from build123d import *

# Parameters (mm, degrees)
SV_DEPTH           = 9
SKETCH3_W          = 35.897762959
SKETCH3_H          = 1.597828601
CUT_EXTRUDE1_DEPTH = 3.5


with BuildPart() as part:
    # Sketch1 → SV (new body)
    with BuildSketch(Plane(origin=(0, 0, 0), x_dir=(1, 0, 0), z_dir=(0, 1, 0))):
        Polygon((-20.189, 2.5), (21.25, 2.5), (21.25, -1.44), (21.25, -2.5), (20.19, -2.5), (-21.25, -2.5), (-21.25, 1.439), align=None)
    extrude(amount=SV_DEPTH)

    # Sketch3 → Cut-Extrude1 (cut)
    with BuildSketch(Plane(origin=(0, 9, 0), x_dir=(1, 0, 0), z_dir=(0, 1, 0))):
        Polygon((-20.202517392, 0.734832739), (-18.867516597, 0.734832739), (-18.867516597, 1.51327079), (19.169882457, 1.51327079), (19.169882457, 0.573528463), (20.36118295, 0.573528463), (20.36118295, -1.024300139), (19.169882457, -1.024300139), (19.169882457, -1.572342426), (-18.867516597, -1.572342426), (-18.867516597, -0.862995862), (-20.202517392, -0.862995862), align=None)
        with Locations((0.304154287, -0.064081561)):
            Rectangle(SKETCH3_W, SKETCH3_H, mode=Mode.SUBTRACT)
    extrude(amount=-CUT_EXTRUDE1_DEPTH, mode=Mode.SUBTRACT)


solid = part.part
Input: part model. Units: mm. Frame: model coordinates. A direction names the side the tool comes from. Round coordinates to 2 decimals unless told otherwise and drop trailing zeros. Write each loop counter-clockwise with the first axis right and the second up, starting at its lowest first coordinate (ties: lowest second). Pieces come first, ordered by that corner, then holes.
1) Cut plane C-C (x = 7). Return the cut outline in (y, z), then the cut area to 3 significant figures.
2) Ray query, L1, parallel to Z at x = 2, y = 5.75; L2, parallel to X at y = 7.75, z = -1.4; L3, parallel to Y at x = -1, z = 1.45. Return the intervals inside material, ascending.
3) Cut plane B-B (z = -0.1). Return the cut outline in (x, y), then the cut area to 3 significant figures.
4) Reachability of faces 1 (the flat face through (20.361, 7, 0)), 2 (the flat face through (0, 4, -2.5)) from +Z, -Z, +X, -X, +Y, -Y: full face, straight path, thin tool, end or side. Return the list, or none.
5) Draft query along X for faces 3 (the flat face through (0, 4, 2.5)), 4 (the flat face through (21.25, 4, 0)), 5 (the flat face through (0, 7, -1.513)). Return one class per face: pulls with the +X half, pulls with the -X half, needs draft (parallel to the pull), parting line crosses it, or undercut.
6) Cut plane A-A (y = 7.75). Return the cut outline in (x, z).
Geometry says:
1. outline: (0, -2.5) - (9, -2.5) - (9, -1.51) - (5.5, -1.51) - (5.5, -0.73) - (9, -0.73) - (9, 0.86) - (5.5, 0.86) - (5.5, 1.57) - (9, 1.57) - (9, 2.5) - (0, 2.5) - close
1. area: 39.8 mm2
2. L1: z = -2.5 to -1.51, -0.73 to 0.86, 1.57 to 2.5
2. L2: x = -21.25 to -18.87, 19.17 to 21.25
2. L3: y = 0 to 5.5
3. outline: (-21.25, 0) - (21.25, 0) - (21.25, 9) - (20.36, 9) - (20.36, 5.5) - (18.25, 5.5) - (18.25, 9) - (-17.64, 9) - (-17.64, 5.5) - (-20.2, 5.5) - (-20.2, 9) - (-21.25, 9) - close
3. area: 366 mm2
4. face 1: +Y
4. face 2: -Z, +X, -X, +Y, -Y
5. face 3: needs draft
5. face 4: pulls with the +X half
5. face 5: undercut
6. outline: (-21.25, -1.44) - (-20.19, -2.5) - (21.25, -2.5) - (21.25, 2.5) - (-21.25, 2.5) - close; (-17.64, -0.73) - (18.25, -0.73) - (18.25, 0.86) - (-17.64, 0.86) - close; hole (-20.2, -0.73) - (-18.87, -0.73) - (-18.87, -1.51) - (19.17, -1.51) - (19.17, -0.57) - (20.36, -0.57) - (20.36, 1.02) - (19.17, 1.02) - (19.17, 1.57) - (-18.87, 1.57) - (-18.87, 0.86) - (-20.2, 0.86) - close
